Part print with two shaded views. Sizes in mm from the minimum x, y, z corner. A direction names the side the tool comes from. Round coordinates to 2 decimals unless told otherwise and drop trailing zeros. Write each loop counter-clockwise with the first axis right and the second up, starting at its lowest first coordinate (ties: lowest second). Pieces come first, ordered by that corner, then holes. Notation, with made-up numbers: (5.5, 3) -> (63.5, 3) arc R21 ccw to (63.5, 35) -> close; hole circle Ø3 at (24.5, 13). An arc over 180 degrees is marked (long way). Answer in a Markdown table with one row per item. Add a question column.
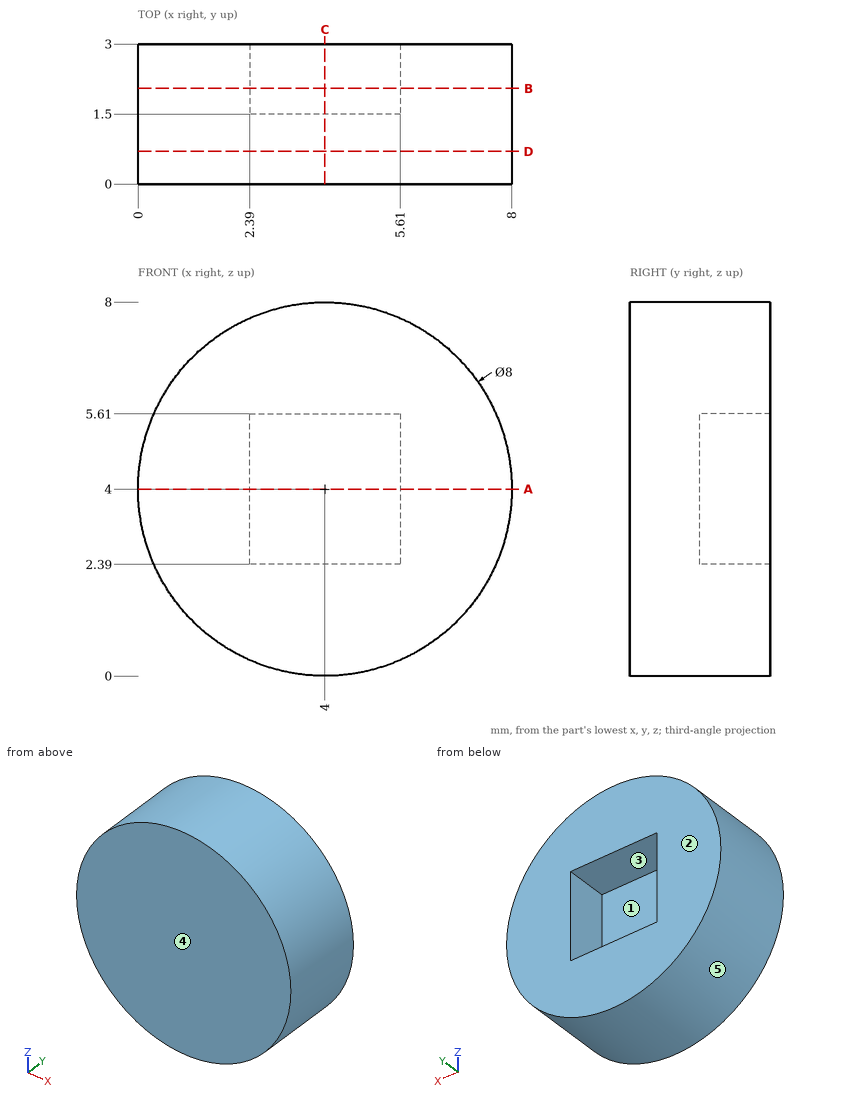
Item 1: Two-plate mould, pull along Z, no slides. Class the marked faces 3, 4 and 5: +Z half, -Z half, draft (parallel to the pull), parting line (faces both ways), or undercut.
Item 2: Saw through at A-A on z = 4. Give the cut face in (x, y), then the cut area to 3 significant figures.
Item 3: Saw through at C-C on x = 4. Give the cut face in (y, z), then the cut area to 3 significant figures.
Item 4: Saw through at B-B on y = 2.05. Give the cut face in (x, z).
Item 5: Tool access for the marked faces 1 and 2: list every direction of +Z, -Z, +X, -X, +Y, -Y with a clear straight run to the whole face (end or side of a thin tool).
Item 6: Drill centre lines: probe 1 along X at (y, z) = (2.95, 5.5); probe 2 along X at (y, z) = (2.7, 3.5); probe 3 along Z at (x, y) = (4.75, 2.8). Where is each one in solid material? Low to high.
Item 7: Saw through at D-D on y = 0.7. Give the cut face in (x, z), then the cut area to 3 significant figures.
Recorded:
| question | item | result |
|---|---|---|
| 1 | face 3 | undercut |
| 1 | face 4 | draft |
| 1 | face 5 | parting line |
| 2 | outline | (0, 0) -> (8, 0) -> (8, 3) -> (5.61, 3) -> (5.61, 1.5) -> (2.39, 1.5) -> (2.39, 3) -> (0, 3) -> close |
| 2 | area | 19.2 mm2 |
| 3 | outline | (0, 0) -> (3, 0) -> (3, 2.39) -> (1.5, 2.39) -> (1.5, 5.61) -> (3, 5.61) -> (3, 8) -> (0, 8) -> close |
| 3 | area | 19.2 mm2 |
| 4 | outline | circle Ø8 at (4, 4); hole (2.39, 2.39) -> (5.61, 2.39) -> (5.61, 5.61) -> (2.39, 5.61) -> close |
| 5 | face 1 | +Y |
| 5 | face 2 | +Z, -Z, +X, -X, +Y |
| 6 | probe 1 | 0.29 to 2.39, 5.61 to 7.71 |
| 6 | probe 2 | 0.03 to 2.39, 5.61 to 7.97 |
| 6 | probe 3 | 0.07 to 2.39, 5.61 to 7.93 |
| 7 | outline | circle Ø8 at (4, 4) |
| 7 | area | 50.3 mm2 |
